Geometry: final body of the model. Coordinates: model frame, mm. A direction names the side the tool comes from. Give positions to 0.01 mm unless a question says otherwise; leave off trailing zeros. Loops run counter-clockwise (first coordinate to the right, second up) from the corner with the lowest first, then second, coordinate; pieces in that order, holes last.
1. Material intervals for line 1 along Z through (x, y) = (0, 143.5); line 2 along X through (y, z) = (136, -7.5); line 3 along X through (y, z) = (142, 0), sorted ascending.
2. First-contact query: P1, Ø4, axis at x = -20, z = 5.5, coming from the -Y side; P2, Ø11, axis at x = 0, z = 0, coming from the -Y side; P3, Ø12, axis at x = 9, z = -7, coming from the -Y side. Flat tips, straight axial feed; report the tip coordinate or a pass-through.
3. Draft query along Z for faces 3 (the face through (0, 2, 10)), 4 (the face through (-1.172, 139.801, -8.923)), 5 (the face through (-30, -2, 0)). Return one class per face: +Z half, -Z half, draft (parallel to the pull), parting line (faces both ways), or undercut.
4. Section C-C, the plane y = 130. Output: boundary loops of the cut face in (x, z), then the cut area to 3 significant figures.
5. Section A-A, the plane x = 0. Output: boundary loops of the cut face in (y, z), then the cut area to 3 significant figures.
6. Access query for faces 1 (the face through (-10.878, 152.958, 0.14)), 2 (the face through (0, 125, 0)). Directions: +Z, -Z, +X, -X, +Y, -Y. A direction counts if a zero-diameter tool reaches every point of the face in a straight line with its end or side. Return the directions, or none.
7. Section B-B, the plane z = 5.5. Output: boundary loops of the cut face in (x, y), then the cut area to 3 significant figures.
8. Section D-D, the plane x = 17. Output: boundary loops of the cut face in (y, z), then the cut area to 3 significant figures.
from build123d import *

# Parameters (mm, degrees)
BOSS_EXTRUDE1_DEPTH = 10
SKETCH5_R           = 9
CUT_EXTRUDE1_DEPTH  = 40


with BuildPart() as part:
    # Sketch3 → Boss-Extrude1 (new body, symmetric)
    with BuildSketch(Plane.XY):
        with BuildLine():
            Line((-30, -125), (-30, 125))
            ThreePointArc((-30, 125), (0, 155), (30, 125))
            Line((30, 125), (30, -125))
            ThreePointArc((30, -125), (0, -155), (-30, -125))
        make_face()
    extrude(amount=BOSS_EXTRUDE1_DEPTH, both=True)

    # Sketch5 → Cut-Extrude1 (cut)
    with BuildSketch(Plane(origin=(0, 125, 0), x_dir=(1, 0, 0), z_dir=(0, 1, 0))):
        Circle(SKETCH5_R)
    extrude(amount=CUT_EXTRUDE1_DEPTH, mode=Mode.SUBTRACT)


solid = part.part
Answers below:
1. line 1: z = -10 to -9, 9 to 10
1. line 2: x = -27.91 to -4.97, 4.97 to 27.91
1. line 3: x = -24.72 to -9, 9 to 24.72
2. P1: stops at y = -149
2. P2: stops at y = -155
2. P3: stops at y = -154.85
3. face 3: +Z half
3. face 4: undercut
3. face 5: draft
4. outline: (-29.58, -10) - (29.58, -10) - (29.58, 10) - (-29.58, 10) - close; hole circle Ø18 at (0, 0)
4. area: 929 mm2
5. outline: (-155, -10) - (155, -10) - (155, -9) - (125, -9) - (125, 9) - (155, 9) - (155, 10) - (-155, 10) - close
5. area: 5,660 mm2
6. face 1: +Z, -Z, +Y
6. face 2: +Y
7. outline: (-30, -125) arc R30 ccw to (30, -125) - (30, 125) arc R30 ccw to (7.12, 154.14) - (7.12, 125) - (-7.12, 125) - (-7.12, 154.14) arc R30 ccw to (-30, 125) - close
7. area: 17,400 mm2
8. outline: (-149.72, -10) - (149.72, -10) - (149.72, 10) - (-149.72, 10) - close
8. area: 5,990 mm2
